from build123d import *

# Parameters (mm, degrees)
F1_DEPTH = 63.5
F2_DEPTH = 25.4
F3_DEPTH = 7.9375
F0_W     = 25.4
F0_H     = 19.05
F4_DEPTH = 25.4
F6_R     = 6.35


# Not quite as in the source:
# - ends of sketch curves that miss each other by under 0.0002 mm in the source are joined
# - a feature names something its author has since deleted; it is built from what else it names


with BuildPart() as f1:
    # F0 (on Front) → F1 (new body, symmetric)
    with BuildSketch(Plane.XZ):
        Polygon((41.275, -9.525), (41.275, 9.525), (22.225, 9.525), (-41.275, 9.525), (-41.275, -9.525), align=None)
    extrude(amount=F1_DEPTH, both=True)

    # F0 (on Front) → F2 (join, symmetric)
    with BuildSketch(Plane.XZ):
        with BuildLine():
            Line((22.225, 9.525), (41.275, 9.525))
            Line((41.275, 9.525), (41.275, 27.0002))
            ThreePointArc((41.275, 27.0002), (45.9246798487, 38.2255201513), (57.15, 42.8752))
            Line((57.15, 42.8752), (68.7916731741, 42.8752))
            Line((68.7916731741, 42.8752), (68.7916731741, 61.9252))
            Line((68.7916731741, 61.9252), (57.15, 61.9252))
            add(Edge.make_bspline(
                [(50.7252492869, 61.329171511), (52.8269652502, 61.534305037), (54.9682888804, 61.732284225), (57.15, 61.9252)],
                knots=[106.8911851376, 106.8911851376, 106.8911851376, 106.8911851376, 111.5045367133, 111.5045367133, 111.5045367133, 111.5045367133], degree=3))
            ThreePointArc((50.7252492869, 61.329171511), (30.2786385449, 49.3090690945), (22.22499883, 27.0002))
            Line((22.22499883, 27.0002), (22.225, 9.525))
        make_face()
    extrude(amount=F2_DEPTH, both=True)

    # F0 (on Front) → F3 (join, symmetric)
    with BuildSketch(Plane.XZ):
        with BuildLine():
            Line((-41.275, 9.525), (22.225, 9.525))
            Line((22.225, 9.525), (22.225, 27.0002))
            ThreePointArc((22.225, 27.0002), (30.2786385449, 49.3090690945), (50.7252492869, 61.329171511))
            add(Edge.make_bspline(
                [(-41.275, 9.525), (-25.4048483065, 47.9825129098), (2.0285682627, 56.5762353117), (50.7252492869, 61.329171511)],
                knots=[0, 0, 0, 0, 106.8911851376, 106.8911851376, 106.8911851376, 106.8911851376], degree=3))
        make_face()
    extrude(amount=F3_DEPTH, both=True)

    # F0 (on Front) → F4 (join, symmetric)
    with BuildSketch(Plane.XZ):
        with Locations((81.4916731741, 52.4002)):
            Rectangle(F0_W, F0_H)
    extrude(amount=F4_DEPTH, both=True)

    # F0 (on Front) → F5 (revolve)
    with BuildSketch(Plane.XZ):
        Polygon((94.1916731741, 61.9252), (94.1916731741, 42.8752), (94.1916731741, 38.1), (119.5916731741, 38.1), (119.5916731741, 66.675), (94.1916731741, 66.675), align=None)
    revolve(axis=Axis((94.1916731741, 0, 52.3875), (0, 0, 1)))

    # F6
    f6_edges = [f1.edges().sort_by_distance(p)[0] for p in [
        (41.275, -63.5, 0),
        (-41.275, -63.5, 0),
        (41.275, 63.5, 0),
        (-41.275, 63.5, 0),
    ]]
    fillet(f6_edges, radius=F6_R)


solid = f1.part
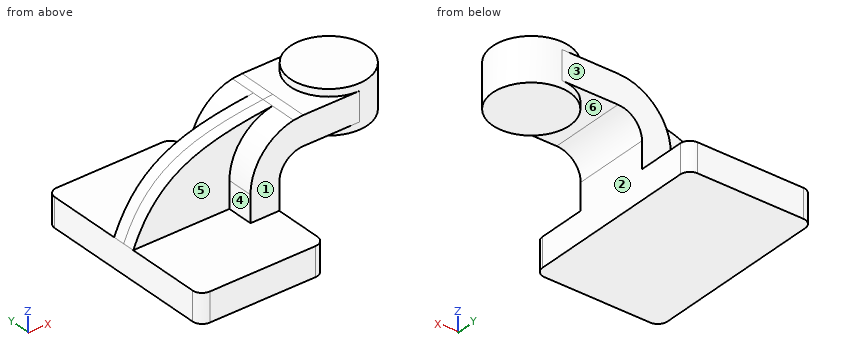
Could you check a few things on this model? Use its own coordinates, in mm. Face numbers are marked on the shaded views. A direction names the side the tool comes from. Round coordinates to 2 decimals unless told otherwise and drop trailing zeros. Loops run counter-clockwise (first coordinate to the right, second up) from the corner with the lowest first, then second, coordinate; pieces in that order, holes last. Notation, with made-up numbers: (9, 44.25) - (61, 44.25) arc R30 cw to (61, 80.25) - close; hole circle Ø3 at (72.25, 59.5). An arc over 180 degrees is marked (long way). Write item = value, one per line.
1) I'm going to push flat-ended pins straight in: P1, Ø15.5, axis at x = 2, z = 38, coming from the +Y side; P2, Ø15.5, axis at x = 68, z = 39, coming from the -Y side; P3, Ø15.5, axis at x = 63, z = 41.5, coming from the +Y side. Where does each tip first touch, or does it pass through?
Computed:
P1 = 7.94
P2 = -25.4
P3 = 25.4
2) Imagine slicing it at B-B (y = 33). Please give me the cut outline in (x, z) (3 decimals), and give its area (3 significant figures).
Computed:
outline = (-41.275, -9.525) - (41.275, -9.525) - (41.275, 9.525) - (-41.275, 9.525) - close
area = 1,570 mm2
3) Imagine slicing it at A-A (x = 74). Please give me the cut outline in (y, z) (3 decimals).
Computed:
outline = (-25.4, 42.875) - (-15.41, 42.875) - (-15.41, 38.1) - (15.41, 38.1) - (15.41, 42.875) - (25.4, 42.875) - (25.4, 61.925) - (15.41, 61.925) - (15.41, 66.675) - (-15.41, 66.675) - (-15.41, 61.925) - (-25.4, 61.925) - close
4) On a 3-axis mill with a long thin cutter (end or side, diameter ignored), from which of +Z, -Z, +X, -X, +Y, -Y can I reach the whole of each face in a straight line? I mean the marked faces 1, 2 and 3. Say none if no direction works.
Computed:
face_1 = +Z, +X, -X, -Y
face_2 = -Z, +X, +Y, -Y
face_3 = +Z, +X, -X, +Y
5) If we mould it in two halves opening along X, with no side actions, what happens to the marked faces 4, 5 and 6? For each: pulls with the +X half, pulls with the -X half, needs draft (parallel to the pull), parting line crosses it, or undercut.
Computed:
face_4 = pulls with the -X half
face_5 = needs draft
face_6 = undercut
6) I need wall thicknesses on line 1 along X through (y, z) = (-23, -6) (3 decimals); line 2 along Y through (x, z) = (34, 33.5); line 3 along Z through (x, y) = (-18, -48) (3 decimals). Which ranges of each line are inside material? Lowest first, please. Write a range as from..to.
Computed:
line_1 = -41.275..41.275
line_2 = -25.4..25.4
line_3 = -9.525..9.525
